Autodesk Inventor part; units mm, degrees
ref_plane "YZ Plane" through (0, 0, 0) normal (1, 0, 0) x (0, 1, 0)
ref_plane "XZ Plane" through (0, 0, 0) normal (0, 1, 0) x (-1, 0, 0)
ref_plane "XY Plane" through (0, 0, 0) normal (0, 0, 1) x (1, 0, 0)
ref_plane "РабПлоскость1" through (-0.858, 10.5846, 17.8317) normal (0, -1, 0) x (1, 0, 0)
ref_plane "РабПлоскость2" through (4.892, 13.1846, 45.3317) normal (0, 1, 0) x (1, 0, 0)
sketch "Эскиз1" plane through (-0.858, 13.1846, 17.8317) normal (0, -1, 0) x (1, 0, 0)
  arc A0 (8.858, -19.8317) -> (11.858, -19.8317) centre (10.358, -20.8267) ccw
  line L0 (8.858, -19.8317) -> (8.858, -17.8317)
  line L1 (11.858, -17.8317) -> (11.858, -19.8317)
  line L2 (11.958, -17.8317) -> (11.958, -21.4012)
  arc A1 (8.958, -21.7911) -> (11.958, -21.4012) centre (10.358, -20.8267) ccw
  line L3 (8.958, -21.7911) -> (8.958, -17.8317)
  line L4 (11.858, -17.8317) -> (13.858, -17.8317)
  line L5 (4.858, -17.8317) -> (8.858, -17.8317)
  line L6 (7.358, -19.8317) -> (7.358, 1.6683)
  line L7 (7.358, 1.6683) -> (-10.642, 1.6683)
  line L8 (-10.642, 1.6683) -> (-10.642, -19.8317)
  line L9 (-12.142, -17.8317) -> (-8.142, -17.8317)
  line L10 (-12.142, -23.8317) -> (-12.142, -17.8317)
  line L11 (13.858, -17.8317) -> (13.858, 5.1683)
  line L12 (13.858, 5.1683) -> (-14.5723, 5.1683)
  line L13 (-14.5723, 5.1683) -> (-14.5723, -25.8317)
  line L14 (-14.5723, -25.8317) -> (-10.142, -25.8317)
  line L15 (-10.142, -25.8317) -> (-10.142, -23.8317)
  line L16 (-12.142, -23.8317) -> (-10.142, -23.8317)
  line L17 (8.858, -17.8317) -> (8.958, -17.8317)
  line L18 (11.858, -17.8317) -> (11.958, -17.8317)
  point P0 (0.858, -17.8317)
  point P1 (-10.642, -17.8317)
  point P2 (7.358, -17.8317)
  point P3 (19.5, 6.5781)
  point P4 (19.5, 4.3408)
  point P5 (1.1058, 1.6683)
  point P6 (19.1666, -17.8317)
  point P7 (11.858, -18.4138)
  point P8 (-4.2637, -11.6345)
  point P9 (-4.2637, 1.6683)
  dimension "d0" = 0.1
  dimension "d1" = 23
  dimension "d2" = 2
  dimension "d3" = 2
extrude "Выдавливание1" add sketch "Эскиз1" against normal blind 15 contours L0 L17 L3 A1 L2 A0 | L2 A1 L3 L17 L5 L6 L7 L8 L9 L10 L16 L15 L14 L13 L12 L11 L4 L1 A0
fillet "Сопряжение1" radius 2 8 edges at (-15.4303, 20.6846, -8) (-15.4303, 13.1846, 7.5) (-15.4303, 28.1846, 7.5) (-15.4303, 20.6846, 23) (-1.2151, 13.1846, 23) (-1.2151, 28.1846, 23) (13, 13.1846, 11.5) (13, 28.1846, 11.5)
properties part number "ЛЦМК.30000.10.00.03 Крышка передняя"
Geometry: final body of the model. Coordinates: model frame, mm. A direction names the side the tool comes from. Give positions to 0.01 mm unless a question says otherwise; leave off trailing zeros. Write each loop counter-clockwise with the first axis right and the second up, starting at its lowest first coordinate (ties: lowest second). Pieces come first, ordered by that corner, then holes. Notation, with made-up numbers: (-4, -5) - (15, -5) arc R37 cw to (15, 33) - close; hole circle Ø9 at (39, 88). An arc over 180 degrees is marked (long way). Return JSON: item names as keys, results as strings. Group by question number.
1) Section D-D on x = -2.25. Return the cut outline in (y, z), plus the area to 3 significant figures.
2) Line query: line 1 (Z direction, x = -11.25, y = 22.75); line 2 (X direction, y = 21, z = -1); line 3 (X direction, y = 17, z = 5). Output: solid intervals per line, ascending.
3) Section A-A on z = 6.5. Return the cut outline in (x, y), plus the area to 3 significant figures.
4) Section B-B on x = 9.5. Return the cut outline in (y, z) (3 decimals), plus the area to 3 significant figures.
5) First-contact query: P1, Ø1, axis at y = 20.5, z = -1, coming from the +X side; P2, Ø7.5, axis at x = 0, y = 21, coming from the -Z side; P3, Ø1, axis at y = 20.5, z = -7, coming from the +X side. Flat tips, straight axial feed; report the tip coordinate or a pass-through.
6) Section C-C on y = 25.5. Return the cut outline in (x, z) (3 decimals).
7) Set-up query: faces 1 (the flat face through (-12, 21, 0)), 2 (the flat face through (-12, 21, -6)), 3 (the flat face through (6.5, 21, 10)). Return all of +Z, -Z, +X, -X, +Y, -Y with unobstructed straight access to the full face (end or side cutting, diameter ignored); none if empty.
Filled in:
{
 "1": {"outline": "(13.18, 19.5) - (28.18, 19.5) - (28.18, 21) arc R2 ccw to (26.18, 23) - (15.18, 23) arc R2 ccw to (13.18, 21) - close", "area": "50.8 mm^2"},
 "2": {"line 1": "z = -8 to -6, 19.5 to 23", "line 2": "x = -15.43 to -13, 8 to 11", "line 3": "x = -15.43 to -11.5, 6.5 to 13"},
 "3": {"outline": "(-15.43, 15.18) arc R2 ccw to (-13.43, 13.18) - (-11.5, 13.18) - (-11.5, 28.18) - (-13.43, 28.18) arc R2 ccw to (-15.43, 26.18) - close; (6.5, 13.18) - (11, 13.18) arc R2 ccw to (13, 15.18) - (13, 26.18) arc R2 ccw to (11, 28.18) - (6.5, 28.18) - close", "area": "153 mm^2"},
 "4": {"outline": "(13.185, -4.795) - (28.185, -4.795) - (28.185, 21) arc R2 ccw to (26.185, 23) - (15.185, 23) arc R2 ccw to (13.185, 21) - close", "area": "415 mm^2"},
 "5": {"P1": "stops at x = 11", "P2": "stops at z = 19.5", "P3": "stops at x = -11"},
 "6": {"outline": "(-15.43, -6) arc R2 ccw to (-13.43, -8) - (-11, -8) - (-11, -6) - (-13, -6) - (-13, 0) - (-11.5, 0) - (-11.5, 19.5) - (6.5, 19.5) - (6.5, 0) - (8, 0) - (8, -2) arc R1.8 ccw (long way) to (11, -2) - (11, 0) - (13, 0) - (13, 23) - (-13.43, 23) arc R2 ccw to (-15.43, 21) - close"},
 "7": {"face 1": "+Y, -Y", "face 2": "+X, +Y, -Y", "face 3": "-Z, +Y, -Y"}
}
